Can you work these out from the model? Positions are in its coordinate system, mm. A direction names the side the tool comes from. Round coordinates to 2 decimals unless told otherwise and drop trailing zeros. Order: outer loops, then holes, each group sorted by start corner. A loop starts at its lowest first (then second) coordinate and runs counter-clockwise, first axis right, second up. Notation, with made-up numbers: (-0.75, 60.5) - (7.25, 60.5) arc R21 cw to (7.25, 67.5) - close; hole circle Ø8 at (22, 1). An arc over 180 degrees is marked (long way). Write item = value, one per line.
from build123d import *

# Parameters (mm, degrees)
BOSS_EXTRUDE1_DEPTH = 4
SKETCH8_R           = 7.4
SKETCH8_R_2         = 5.000519882
BOSS_EXTRUDE2_DEPTH = 4
SKETCH9_W           = 74.744017839
SKETCH9_H           = 24
BOSS_EXTRUDE3_DEPTH = 4
FILLET1_R           = 4.5
FILLET2_R           = 3
SKETCH10_R          = 2.1
CUT_EXTRUDE1_DEPTH  = 128.760117479


with BuildPart() as part:
    # Sketch3 → Boss-Extrude1 (new body)
    with BuildSketch(Plane.XY.offset(-7.75)):
        with BuildLine():
            Line((-1.659393939, 7.211547112), (-33, 0))
            ThreePointArc((-33, 0), (-44.924936548, 4.974434641), (-40.07, -6.999649991))
            Line((-40.07, -6.999649991), (-0.074, -7.399629991))
            ThreePointArc((-0.074, -7.399629991), (0.036988131, -7.399907559), (0.147967941, -7.398520493))
            Line((0.147967941, -7.398520493), (120.099988734, -4.999520111))
            ThreePointArc((120.099988734, -4.999520111), (125.000519882, 0), (120.099988734, 4.999520111))
            Line((120.099988734, 4.999520111), (0.147967941, 7.398520493))
            ThreePointArc((0.147967941, 7.398520493), (-0.761473505, 7.360717227), (-1.659393939, 7.211547112))
        make_face()
    extrude(amount=-BOSS_EXTRUDE1_DEPTH)



with BuildPart() as body_2:
    # Sketch8 → Boss-Extrude2 (new body)
    with BuildSketch(Plane(origin=(0, 0, -27.75), x_dir=(-1, 0, 0), z_dir=(0, 0, -1))):
        Circle(SKETCH8_R)
        with BuildLine():
            Line((-120.099988734, -4.999520111), (-0.147967941, -7.398520493))
            ThreePointArc((-0.147967941, -7.398520493), (-7.4, 0), (-0.147967941, 7.398520493))
            Line((-0.147967941, 7.398520493), (-120.099988734, 4.999520111))
            ThreePointArc((-120.099988734, 4.999520111), (-116.499628346, 3.5710779), (-114.999480118, 0))
            ThreePointArc((-114.999480118, 0), (-116.499628346, -3.5710779), (-120.099988734, -4.999520111))
        make_face()
        with Locations((-120, 0)):
            Circle(SKETCH8_R_2)
    extrude(amount=BOSS_EXTRUDE2_DEPTH)


with BuildPart() as part_1:
    add(part.part)

    add(body_2.part)  # Boss-Extrude3 merges body 2
    # Sketch9 → Boss-Extrude3 (add)
    with BuildSketch(Plane(origin=(0.147967941, 7.398520493, 0), x_dir=(0.999800066650892, -0.019995667652563644, 0), z_dir=(0.019995667652563644, 0.999800066650892, 0))):
        with Locations((56.086957222, 19.75)):
            Rectangle(SKETCH9_W, SKETCH9_H)
    extrude(amount=BOSS_EXTRUDE3_DEPTH)

    # Fillet1
    fillet1_edges = [part_1.edges().sort_by_distance(p)[0] for p in [
        (56.30369418, 10.276224604, -7.75),
        (56.30369418, 10.276224604, -31.75),
    ]]
    fillet(fillet1_edges, radius=FILLET1_R)

    # Fillet2
    fillet2_edges = [part_1.edges().sort_by_distance(p)[0] for p in [
        (18.8591745, 7.024302607, -9.763932023),
        (93.588248518, 5.529746067, -29.736067977),
        (93.588248518, 5.529746067, -9.763932023),
        (18.8591745, 7.024302607, -29.736067977),
    ]]
    fillet(fillet2_edges, radius=FILLET2_R)

    # Sketch10 → Cut-Extrude1 (cut, through all)
    with BuildSketch(Plane.XY.offset(-7.75)):
        with Locations((-40, 0)):
            Circle(SKETCH10_R)
        Circle(SKETCH10_R)
        with Locations((120, 0)):
            Circle(SKETCH10_R)
    extrude(amount=-CUT_EXTRUDE1_DEPTH, mode=Mode.SUBTRACT)


solid = part_1.part
(1) If we section it at A-A (y = -3.5): Write out the boundary of the cut face in (x, z).
Computed:
outline = (-46.06, -11.75) - (123.57, -11.75) - (123.57, -7.75) - (-46.06, -7.75) - close; (-6.52, -31.75) - (123.57, -31.75) - (123.57, -27.75) - (-6.52, -27.75) - close
(2) Will these pins go through, and if not, where does the flat tip stop? P1, Ø8, axis at x = -26, y = -1.5, coming from the -Z side; P2, Ø6, axis at y = 5, z = -18.5, coming from the -X side; P3, Ø1, axis at y = 6, z = -22, coming from the +X side.
Computed:
P1 = -11.75
P2 = 18.86
P3 = 93.61
(3) If we section it at B-B (z = -25.75): Write out the boundary of the cut face in (x, y).
Computed:
outline = (18.86, 7.02) - (93.59, 5.53) - (93.67, 9.53) - (18.94, 11.02) - close
(4) Thinking about a two-plate mould opening in Y: for faces 4 (the face through (2.003, 0.631, -29.722)), 5 (the face through (58, 0, -31.75)), 6 (the face through (-17.11, 3.656, -9.722)), which applies, +Y half, -Y half, draft (parallel to the pull), parting line (faces both ways), or undercut?
Computed:
face_4 = undercut
face_5 = draft
face_6 = +Y half
(5) If I drill on line 1 (Y direction, x = -40, z = -9.8); line 2 (Z direction, x = 101.5, y = 2.5); line 3 (Y direction, x = 0, z = -10.15), over which ranges is the centre line in solid material (lowest first)? Write a range as from..to.
Computed:
line_1 = -7..-2.1, 2.1..7
line_2 = -31.75..-27.75, -11.75..-7.75
line_3 = -7.4..-2.1, 2.1..7.4
(6) On a 3-axis mill with a long thin cutter (end or side, diameter ignored), from which of +Z, -Z, +X, -X, +Y, -Y can I reach the whole of each face in a straight line? I mean faces 1 (the face through (18.02, 7.94, -29.76)), 2 (the face through (60.7, 8.8, -9)), 3 (the face through (-42.1, 0.09, -9.72)). Say none if no direction works.
Computed:
face_1 = +Z, -Z, +Y
face_2 = +Z, +X, +Y
face_3 = +Z, -Z
